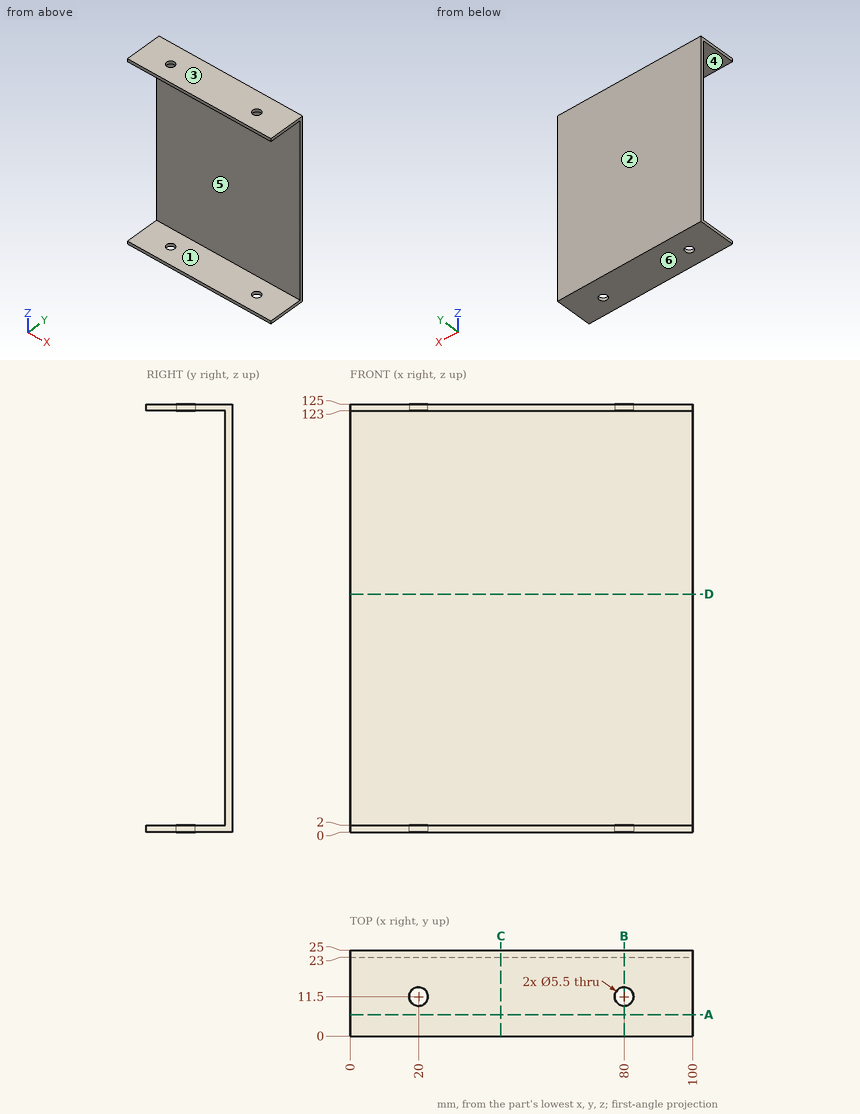
Verification items for this drawing (mm, ordinates from the low corner). A direction names the side the tool comes from. Round coordinates to 2 decimals unless told otherwise and drop trailing zeros. Loops run counter-clockwise (first coordinate to the right, second up) from the corner with the lowest first, then second, coordinate; pieces in that order, holes last. Notation, with made-up numbers: (69.25, -1.75) - (118.25, -1.75) arc R33 ccw to (118.25, 34.25) - close; hole circle Ø10 at (61.25, 81.25). An arc over 180 degrees is marked (long way). Answer as CSV lines item,"result". Start each with the question number.
Item 1: Set-up check for the marked faces 1 and 2: record each of +Z, -Z, +X, -X, +Y, -Y from which the full face is reachable in a straight line by a thin tool's end or side.
Item 2: Section check D-D (z = 69.5). Record the boundary of the cut face in (x, y).
Item 3: Section check C-C (x = 44). Record the boundary of the cut face in (y, z).
Item 4: Section check B-B (x = 80). Record the boundary of the cut face in (y, z).
Item 5: Scan lines: line 1 (X direction, y = 11.5, z = 124.4); line 2 (Z direction, x = 88, y = 14.5); line 3 (Y direction, x = 80, z = 124). Record each from-to range of solid material in increasing order. Write a range as [from, to].
Item 6: Release check for a two-part mould opening along Z. For the marked faces 3, 4, 5 and 6 record: +Z half, -Z half, draft (parallel to the pull), parting line (faces both ways), or undercut.
Item 7: Section check A-A (y = 6.25). Record the boundary of the cut face in (x, z), and give its area (3 significant figures).
Item 8: Depth check by flat-ended pin: P1, Ø4.5, axis at x = 20, y = 11.5, coming from the +Z side; P2, Ø5, axis at x = 68.5, z = 33, coming from the -Y side. Enter the tip coordinate at first touch or a pass-through.
Report:
1,face 1,"+X, -X, -Y"
1,face 2,"+Z, -Z, +X, -X, +Y"
2,outline,"(0, 23) - (100, 23) - (100, 25) - (0, 25) - close"
3,outline,"(0, 0) - (25, 0) - (25, 125) - (0, 125) - (0, 123) - (23, 123) - (23, 2) - (0, 2) - close"
4,outline,"(0, 0) - (8.75, 0) - (8.75, 2) - (0, 2) - close; (0, 123) - (8.75, 123) - (8.75, 125) - (0, 125) - close; (14.25, 0) - (25, 0) - (25, 125) - (14.25, 125) - (14.25, 123) - (23, 123) - (23, 2) - (14.25, 2) - close"
5,line 1,"x = [0, 17.25], [22.75, 77.25], [82.75, 100]"
5,line 2,"z = [0, 2], [123, 125]"
5,line 3,"y = [0, 8.75], [14.25, 25]"
6,face 3,"+Z half"
6,face 4,"undercut"
6,face 5,"undercut"
6,face 6,"-Z half"
7,outline,"(0, 0) - (100, 0) - (100, 2) - (0, 2) - close; (0, 123) - (100, 123) - (100, 125) - (0, 125) - close"
7,area,"400 mm2"
8,P1,"passes through"
8,P2,"stops at y = 23"
